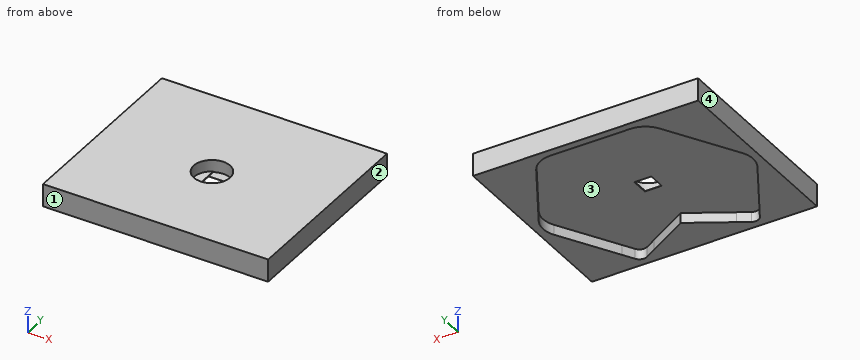
Autodesk Inventor part; units mm, degrees
ref_plane "YZ Plane" through (0, 0, 0) normal (1, 0, 0) x (0, 1, 0)
ref_plane "XZ Plane" through (0, 0, 0) normal (0, 1, 0) x (-1, 0, 0)
ref_plane "XY Plane" through (0, 0, 0) normal (0, 0, 1) x (1, 0, 0)
sketch "Sketch1" plane through (0, 0, 0) normal (0, 0, 1) x (1, 0, 0)
  line L0 (-27.3013, -27.7128) -> (-40.4145, -5)
  line L1 (-40.4145, 5) -> (-24.5374, 32.5)
  line L2 (-15.8771, 37.5) -> (15.8771, 37.5)
  line L3 (24.5374, 32.5) -> (40.4145, 5)
  line L4 (40.4145, -5) -> (27.3013, -27.7128)
  line L5 (21.6506, -37.5) -> (-21.6506, -37.5)
  line L6 (16.3731, -30.641) -> (0, -21.188)
  line L7 (0, -21.188) -> (-16.3731, -30.641)
  circle A0 centre (0, 0) radius 4.75
  line L8 (43.3013, 0) -> (41.7543, 0)
  arc A1 (20.7032, -33.141) -> (24.8013, -32.0429) centre (22.2032, -30.5429) ccw
  arc A2 (-24.8013, -32.0429) -> (-20.7032, -33.141) centre (-22.2032, -30.5429) ccw
  arc A3 (40.4145, -5) -> (40.4145, 5) centre (31.7543, 0) ccw
  arc A4 (24.5374, 32.5) -> (15.8771, 37.5) centre (15.8771, 27.5) ccw
  arc A5 (-15.8771, 37.5) -> (-24.5374, 32.5) centre (-15.8771, 27.5) ccw
  arc A6 (-40.4145, 5) -> (-40.4145, -5) centre (-31.7543, 0) ccw
  circle A7 centre (0, 0) radius 3.375
  line L9 (0, -21.188) -> (0, -37.5)
  circle A8 centre (0, 0) radius 7.225
  line L10 (0, 0) -> (-7.225, 0)
  line L11 (-9.225, 0) -> (-9.225, -16.1218)
  line L12 (-19.2032, -35.7391) -> (0, -24.6521)
  line L13 (0, -24.6521) -> (19.2032, -35.7391)
  arc A9 (19.2032, -35.7391) -> (27.3993, -33.5429) centre (22.2032, -30.5429) ccw
  line L14 (27.3993, -33.5429) -> (43.0126, -6.5)
  arc A10 (43.0126, -6.5) -> (43.0126, 6.5) centre (31.7543, 0) ccw
  line L15 (43.0126, 6.5) -> (27.1355, 34)
  arc A11 (27.1355, 34) -> (15.8771, 40.5) centre (15.8771, 27.5) ccw
  line L16 (15.8771, 40.5) -> (-15.8771, 40.5)
  arc A12 (-15.8771, 40.5) -> (-27.1355, 34) centre (-15.8771, 27.5) ccw
  line L17 (-27.1355, 34) -> (-43.0126, 6.5)
  arc A13 (-43.0126, 6.5) -> (-43.0126, -6.5) centre (-31.7543, 0) ccw
  line L18 (-43.0126, -6.5) -> (-27.3993, -33.5429)
  arc A14 (-27.3993, -33.5429) -> (-19.2032, -35.7391) centre (-22.2032, -30.5429) ccw
  line L19 (-15.225, -22.1218) -> (-16.1451, -22.1218)
  line L20 (-22.1451, -16.1218) -> (-22.1451, 22.5)
  line L21 (-14.1451, 30.5) -> (0, 30.5)
  arc A15 (-14.1451, 30.5) -> (-22.1451, 22.5) centre (-14.1451, 22.5) ccw
  arc A16 (-22.1451, -16.1218) -> (-16.1451, -22.1218) centre (-16.1451, -16.1218) ccw
  arc A17 (-15.225, -22.1218) -> (-9.225, -16.1218) centre (-15.225, -16.1218) ccw
  line L22 (0, 0) -> (0, 30.5)
  line L23 (9.225, 0) -> (9.225, -16.1218)
  arc A18 (9.225, -16.1218) -> (15.225, -22.1218) centre (15.225, -16.1218) ccw
  line L24 (15.225, -22.1218) -> (16.1451, -22.1218)
  arc A19 (16.1451, -22.1218) -> (22.1451, -16.1218) centre (16.1451, -16.1218) ccw
  line L25 (22.1451, -16.1218) -> (22.1451, 22.5)
  arc A20 (22.1451, 22.5) -> (14.1451, 30.5) centre (14.1451, 22.5) ccw
  line L26 (14.1451, 30.5) -> (0, 30.5)
  circle A21 centre (0, 0) radius 9.225
  line L27 (-22.2032, -30.5429) -> (-24.8013, -32.0429)
  line L28 (-22.2032, -30.5429) -> (-20.7032, -33.141)
  line L29 (22.2032, -30.5429) -> (20.7032, -33.141)
  line L30 (22.2032, -30.5429) -> (24.8013, -32.0429)
  arc A22 (-25.8013, -30.3109) -> (-28.3993, -31.8109) centre (-27.1003, -31.0609) ccw
  arc A23 (-17.4711, -34.7391) -> (-18.9711, -32.141) centre (-18.2211, -33.4401) ccw
  arc A24 (28.3993, -31.8109) -> (25.8013, -30.3109) centre (27.1003, -31.0609) ccw
  arc A25 (18.9711, -32.141) -> (17.4711, -34.7391) centre (18.2211, -33.4401) ccw
  line L31 (-14.1451, 30.5) -> (-25.6921, 30.5)
  line L32 (14.1451, 30.5) -> (25.6921, 30.5)
  line L33 (-16.1451, -22.1218) -> (-30.5293, -22.1218)
  line L34 (16.1451, -22.1218) -> (30.5293, -22.1218)
  line L35 (24.8013, -32.0429) -> (40.4145, -5)
  arc A26 (40.4145, -5) -> (40.4145, 5) centre (31.7543, 0) ccw
  line L36 (40.4145, 5) -> (24.5374, 32.5)
  arc A27 (24.5374, 32.5) -> (15.8771, 37.5) centre (15.8771, 27.5) ccw
  line L37 (15.8771, 37.5) -> (-15.8771, 37.5)
  arc A28 (-15.8771, 37.5) -> (-24.5374, 32.5) centre (-15.8771, 27.5) ccw
  line L38 (-24.5374, 32.5) -> (-40.4145, 5)
  arc A29 (-40.4145, 5) -> (-40.4145, -5) centre (-31.7543, 0) ccw
  line L39 (-40.4145, -5) -> (-24.8013, -32.0429)
  arc A30 (20.7032, -33.141) -> (24.8013, -32.0429) centre (22.2032, -30.5429) ccw
  line L40 (20.7032, -33.141) -> (0, -21.188)
  line L41 (0, -21.188) -> (-20.7032, -33.141)
  arc A31 (-24.8013, -32.0429) -> (-20.7032, -33.141) centre (-22.2032, -30.5429) ccw
  line L42 (27.8503, -29.7619) -> (27.8503, -29.7619)
  line L43 (16.9221, -32.6901) -> (16.9221, -32.6901)
  line L44 (-16.9221, -32.6901) -> (-16.9221, -32.6901)
  line L45 (-27.8503, -29.7619) -> (-27.8503, -29.7619)
  arc A32 (27.3013, -27.7128) -> (27.8503, -29.7619) centre (28.6003, -28.4628) ccw
  arc A33 (16.9221, -32.6901) -> (16.3731, -30.641) centre (15.6231, -31.9401) ccw
  arc A34 (-16.3731, -30.641) -> (-16.9221, -32.6901) centre (-15.6231, -31.9401) ccw
  arc A35 (-27.8503, -29.7619) -> (-27.3013, -27.7128) centre (-28.6003, -28.4628) ccw
  line L46 (-24.5374, 32.5) -> (-21.6506, 37.5)
  line L47 (-15.8771, 37.5) -> (-21.6506, 37.5)
  line L48 (15.8771, 37.5) -> (21.6506, 37.5)
  line L49 (24.5374, 32.5) -> (21.6506, 37.5)
  line L50 (30.1451, -22.7872) -> (30.1451, 22.7872)
  line L51 (-30.1451, -22.7872) -> (-30.1451, 22.7872)
  line L52 (-44.7543, 40.5) -> (44.7543, 40.5)
  line L53 (44.7543, 40.5) -> (44.7543, -36.5429)
  line L54 (44.7543, -36.5429) -> (-44.7543, -36.5429)
  line L55 (-44.7543, -36.5429) -> (-44.7543, 40.5)
  line L56 (-3.375, 6.3883) -> (-3.375, -6.3883)
  line L57 (3.375, 6.3883) -> (3.375, -6.3883)
  line L58 (-6.3883, 3.375) -> (6.3883, 3.375)
  line L59 (-6.3883, -3.375) -> (6.3883, -3.375)
  point P0 (-43.3013, 0)
  point P1 (36.8061, -2.25)
  point P2 (6.0982, -2.25)
  point P3 (19.9965, -30.1349)
  point P4 (4.9976, -4.1562)
  point P5 (-6.0982, 2.25)
  point P6 (-36.8061, 2.25)
  point P7 (-36.8061, -2.25)
  point P8 (-6.0982, -2.25)
  point P9 (-20.3516, 30.75)
  point P10 (-4.9976, 4.1562)
  point P11 (-1.1005, 6.4062)
  point P12 (-16.4545, 33)
  point P13 (16.4545, 33)
  point P14 (1.1005, 6.4062)
  point P15 (4.9976, 4.1562)
  point P16 (20.3516, 30.75)
  point P17 (36.8061, 2.25)
  point P18 (6.0982, 2.25)
  point P19 (1.1005, -6.4062)
  point P20 (12.2023, -25.6349)
  point P21 (-4.9976, -4.1562)
  point P22 (-19.9965, -30.1349)
  point P23 (-12.2023, -25.6349)
  point P24 (-1.1005, -6.4062)
  point P25 (-9.225, -26.5141)
  point P26 (7, 0)
  point P27 (0, 7.225)
  point P28 (17.4711, -34.7391)
  point P29 (28.3993, -31.8109)
  point P30 (25.8013, -30.3109)
  point P31 (24.8013, -32.0429)
  point P32 (20.7032, -33.141)
  point P33 (18.9711, -32.141)
  point P34 (-20.7032, -33.141)
  point P35 (-24.8013, -32.0429)
  point P36 (30.1451, -22.1218)
  point P37 (30.1451, 22.7872)
  point P38 (-30.1451, 22.7872)
  point P39 (-30.1451, -22.1218)
  point P40 (-27.8503, -29.7619)
  point P41 (-16.9221, -32.6901)
  point P42 (27.8503, -29.7619)
  point P43 (15.8771, 40.5)
  point P44 (27.3013, -27.7128)
  point P45 (3.375, 3.375)
  point P46 (-3.375, 3.375)
  point P47 (-3.375, -3.375)
  point P48 (3.375, -3.375)
  dimension "d11" = 14.45
  dimension "d0" = 9.5
  dimension "d1" = 120
  dimension "d2" = 75
  dimension "d3" = 40
  dimension "d4" = 3
  dimension "d5" = 10
  dimension "d6" = 6.75
  dimension "d7" = 3
  dimension "d8" = 8
  dimension "d9" = 6
  dimension "d10" = 6
  dimension "d12" = 2
  dimension "d13" = 2
  dimension "d14" = 2
  dimension "d15" = 6
  dimension "d16" = 0
  dimension "d17" = 0
  dimension "d18" = 0
  dimension "d19" = 0
  dimension "d20" = 0
  dimension "d21" = 1.5
  dimension "d22" = 7
  dimension "d23" = 8
extrude "Extrusion1" add sketch "Sketch1" along normal blind 5 contours A35 A22 L18 A13 L17 A12 L16 A11 L15 A10 L14 A24 A32 L4 A3 L3 L49 L48 L2 L47 L46 L1 A6 L0 | L0 L51 L33 L19 A17 L11 A21 L23 A18 L24 L34 L50 L4 L35 L30 L29 L40 L6 L7 L41 L28 L27 L39 | L39 A22 A35 | L0 L33 L51 | L39 A2 L41 A23 L12 A14 L18 A22 | L0 A6 L1 L51 L33 | L51 L1 L31 A15 L20 A16 L33 | L27 L28 A2 | L18 A14 L54 L55 A13 | A16 L20 A15 L21 L22 A21 L11 A17 L19 | L1 A5 L2 A4 L3 L32 L26 L21 L31 | L41 A34 A23 | L55 L52 A12 L17 A13 | A14 L12 L9 L54 | L46 L47 A5 | A34 L7 L9 L12 A23 | L9 L13 A9 L54 | A8 L57 L58 A0 L22 | L22 A0 L58 L56 A8 | A21 | L26 A20 L25 A19 L24 A18 L23 A21 L22 | L6 A33 A25 L13 L9 | A9 L13 A25 L40 A1 L35 A24 L14 | A9 L14 A10 L53 L54 | L48 L49 A4 | L32 L3 L50 L34 A19 L25 A20 | L40 A25 A33 | L52 L53 A10 L15 A11 | A8 L58 L57 | L56 L58 A8 | L22 L58 A0 | A0 L58 L22 | L3 A3 L4 L34 L50 | L29 L30 A1 | A24 L35 A32 | A8 L59 L57 A0 L58 | L57 A0 L58 | L58 L56 A0 L10 A8 | L58 A0 L56 | A0 L57 A7 L58 | L58 A7 L56 A0 | L22 L10 A7 | A7 L10 L22 | L34 L4 L50 | A0 L57 | L10 A0 L56 L59 A8 | L56 L10 A0 | L57 A0 L59 A7 | L56 A0 L10 | A7 L59 A0 L56 | A8 L57 L59 | L59 L56 A8 | L59 A0 | L57 L59 A0 | A0 L59 L56 | A8 L56 L59 A0 L57
extrude "Extrusion2" add sketch "Sketch1" against normal blind 4 contours A35 A22 L18 A13 L17 A12 L16 A11 L15 A10 L14 A24 A32 L4 A3 L3 L49 L48 L2 L47 L46 L1 A6 L0 | L39 A22 A35 | L39 A2 L41 A23 L12 A14 L18 A22 | L18 A14 L54 L55 A13 | L41 A34 A23 | L55 L52 A12 L17 A13 | A14 L12 L9 L54 | L46 L47 A5 | A34 L7 L9 L12 A23 | L9 L13 A9 L54 | L6 A33 A25 L13 L9 | A9 L13 A25 L40 A1 L35 A24 L14 | A9 L14 A10 L53 L54 | L48 L49 A4 | L40 A25 A33 | L52 L53 A10 L15 A11 | A24 L35 A32
extrude "Extrusion3" cut sketch "Sketch1" along normal through all contours A8 L57 L58 A0 L22 | L22 A0 L58 L56 A8 | A8 L58 L57 | L56 L58 A8 | L22 L58 A0 | A0 L58 L22 | A8 L59 L57 A0 L58 | L57 A0 L58 | L58 L56 A0 L10 A8 | L58 A0 L56 | A0 L57 A7 L58 | L58 A7 L56 A0 | L22 L10 A7 | A7 L10 L22 | A0 L57 | L10 A0 L56 L59 A8 | L56 L10 A0 | L57 A0 L59 A7 | L56 A0 L10 | A7 L59 A0 L56 | A8 L57 L59 | L59 L56 A8 | L59 A0 | L57 L59 A0 | A0 L59 L56 | A8 L56 L59 A0 L57
extrude "Extrusion5" add sketch "Sketch1" along normal blind 0.35 contours A8 L58 L57 | L56 L58 A8 | A8 L59 L57 A0 L58 | L58 L56 A0 L10 A8 | A0 L57 | L10 A0 L56 L59 A8 | L56 L10 A0 | L56 A0 L10 | A8 L57 L59 | L59 L56 A8
extrude "Extrusion6" add sketch "Sketch1" along normal blind 0.1 contours A8 L57 L58 A0 L22 | L22 A0 L58 L56 A8 | L22 L58 A0 | A0 L58 L22 | L59 A0 | A8 L56 L59 A0 L57
properties part number "CalibrationBlockV3"
Work out the finished part from the listing and answer in its coordinate system (mm). Face numbers are marked on the shaded views. Give positions to 0.01 mm unless a question says otherwise; leave off trailing zeros. Loops run counter-clockwise (first coordinate to the right, second up) from the corner with the lowest first, then second, coordinate; pieces in that order, holes last. Notation, with made-up numbers: (5.5, 9) -> (29.5, 9) arc R14 cw to (29.5, 19) -> close; hole circle Ø4 at (-12.5, 62). An arc over 180 degrees is marked (long way). Use CSV: the item, a comma, the result in double quotes.
1. Straight lines are drawn through the part: line 1 (X direction, y = 0, z = 1.15) (3 decimals); line 2 (Y direction, x = 0, z = 2.55) (3 decimals); line 3 (Z direction, x = 19, y = 18.5). For each, find the intervals that lie inside material, in ascending order.
Found:
line 1,"-44.754 to -7.225, 7.225 to 44.754"
line 2,"-36.543 to -7.225, 7.225 to 40.5"
line 3,"0 to 5"
2. Flat-ended cylindrical pins translate along their axes: pin 1 Ø4 at (x, y) = (0, -5) entering from +Z; pin 2 Ø4 at (x, y) = (6, 0) entering from +Z; pin 3 Ø1.2 at (x, y) = (-5.5, -0.5) entering from +Z. Find the tip coordinate at first contact, or state that the pin passes through.
Found:
pin 1,"z = 0.1"
pin 2,"z = 5"
pin 3,"z = 0.35"
3. The part is cut by section A-A (y = 0). Write down the section's boundary in (x, z) (3 decimals).
Found:
outline,"(-44.754, -4) -> (-41.754, -4) -> (-41.754, 0) -> (-3.375, 0) -> (-3.375, 0.35) -> (-7.225, 0.35) -> (-7.225, 5) -> (-44.754, 5) -> close; (3.375, 0) -> (41.754, 0) -> (41.754, -4) -> (44.754, -4) -> (44.754, 5) -> (7.225, 5) -> (7.225, 0.35) -> (3.375, 0.35) -> close"
4. The part is cut by section C-C (x = 35). Write down the section's boundary in (y, z), then the cut area to 3 significant figures.
Found:
outline,"(-36.54, -4) -> (-14.38, -4) -> (-14.38, 0) -> (14.38, 0) -> (14.38, -4) -> (40.5, -4) -> (40.5, 5) -> (-36.54, 5) -> close"
area,"578 mm^2"
5. The mould has two halves that part along X. Classify the marked faces 1, 2, 3 and 4: +X half, -X half, draft (parallel to the pull), parting line (faces both ways), or undercut.
Found:
face 1,"draft"
face 2,"+X half"
face 3,"undercut"
face 4,"-X half"
6. The part is cut by section D-D (y = -14). Write down the section's boundary in (x, z), then the cut area to 3 significant figures.
Found:
outline,"(-44.75, -4) -> (-35.22, -4) -> (-35.22, 0) -> (35.22, 0) -> (35.22, -4) -> (44.75, -4) -> (44.75, 5) -> (-44.75, 5) -> close"
area,"524 mm^2"
7. The part is cut by section B-B (z = 4). Write down the section's boundary in (x, y) (3 decimals), then the cut area to 3 significant figures.
Found:
outline,"(-44.754, -36.543) -> (44.754, -36.543) -> (44.754, 40.5) -> (-44.754, 40.5) -> close; hole circle Ø14.45 at (0, 0)"
area,"6,730 mm^2"
